Build history of the part. All positions in model axes, mm. A direction names the side the tool comes from. Give positions to 0.01 mm unless a question says otherwise; leave off trailing zeros. Loops run counter-clockwise (first coordinate to the right, second up) from the corner with the lowest first, then second, coordinate; pieces in that order, holes last. Notation, with made-up numbers: (84, 85.25) -> (89, 85.25) arc R23 cw to (89, 124.25) -> close; hole circle Ø2 at (7.25, -17.75). An arc over 180 degrees is marked (long way). One line per question, with ' | ' between items. Start each with the question number.
(1) Flat gauge pins, fed straight in: pin 1 Ø5 at (y, z) = (-27.5, 126.5) entering from +X; pin 2 Ø1 at (x, z) = (-9.5, 86.5) entering from +Y; pin 3 Ø1 at (x, z) = (6, 26.5) entering from -Y; pin 4 Ø21.5 at (x, y) = (0, 0) entering from -Z. Where does each tip first touch, or does it go through?
(2) Drill centre lines: L1, parallel to Y at x = 0, z = 6; L2, parallel to Z at x = -7.5, y = 23.5; L3, parallel to X at y = -15.5, z = 70.5. Where is each one in solid material? Low to high. Write a range as from..to.
(3) Slice it at C-C, the plane z = 54. Write the cut outline in (x, y), then the cut area to 3 significant figures.
(4) Mould opens along X. For faces 1 (the face through (-1, -10, 0)), 2 (the face through (-2.798, 8.885, 10.14)), 3 (the face through (47.69, -15.02, 51.76)) say: pulls with the +X half, pulls with the -X half, needs draft (parallel to the pull), parting line crosses it, or undercut.
(5) Slice it at B-B, the plane y = 41. Write the cut outline in (x, z), then the cut area to 3 significant figures.
(6) Slice it at A-A, the plane x = -43. Write the cut outline in (y, z), then the cut area to 3 significant figures.
(7) 3-axis set-ups, long thin cutter, end or side, ignore diameter. For faces 4 (the face through (0, 0, 150)), 5 (the face through (10, 11, 130)): which of +Z, -Z, +X, -X, +Y, -Y reach the whole face in a straight line?
Autodesk Inventor part; units mm, degrees
ref_plane "YZ Plane" through (0, 0, 0) normal (1, 0, 0) x (0, 1, 0)
ref_plane "XZ Plane" through (0, 0, 0) normal (0, 1, 0) x (-1, 0, 0)
ref_plane "XY Plane" through (0, 0, 0) normal (0, 0, 1) x (1, 0, 0)
sketch "Sketch1" plane through (0, 0, 0) normal (0, 1, 0) x (-1, 0, 0)
  line L0 (0, 0) -> (0, 150)
  line L1 (0, 150) -> (-14, 150)
  line L2 (-14, 150) -> (-14, 130)
  line L3 (-14, 130) -> (-47.5, 130)
  line L4 (-47.5, 130) -> (-47.5, 105)
  line L5 (-47.5, 105) -> (-50, 105)
  line L6 (-50, 105) -> (-50, 0)
  line L7 (-50, 0) -> (0, 0)
  dimension "d0" = 20
  dimension "d1" = 130
  dimension "d2" = 95
  dimension "d3" = 100
  dimension "d4" = 25
  dimension "d5" = 28
revolve "Revolution1" add sketch "Sketch1" angle 360 about axis through (0, 0, 0) along (0, 0, 1)
sketch "Sketch2" plane through (0, 0, 0) normal (0, 0, -1) x (-1, 0, 0)
  point P0 (0, 0)
hole "Hole1" at (0, 0, 0) direction (0, 0, 1) diameter 18.631 depth 20 tip angle 118
properties part number "Pulse compensator"
Final values:
1) pin 1: x = 40.39 | pin 2: y = 49.18 | pin 3: y = -49.7 | pin 4: z = 0
2) L1: -50..-9.32, 9.32..50 | L2: 0..130 | L3: -47.54..47.54
3) outline: circle Ø100 at (0, 0) | area: 7,850 mm2
4) face 1: needs draft | face 2: undercut | face 3: parting line crosses it
5) outline: (-28.62, 0) -> (28.62, 0) -> (28.62, 105) -> (23.98, 105) -> (23.98, 130) -> (-23.98, 130) -> (-23.98, 105) -> (-28.62, 105) -> close | area: 7,210 mm2
6) outline: (-25.51, 0) -> (25.51, 0) -> (25.51, 105) -> (20.18, 105) -> (20.18, 130) -> (-20.18, 130) -> (-20.18, 105) -> (-25.51, 105) -> close | area: 6,370 mm2
7) face 4: +Z, +X, -X, +Y, -Y | face 5: +Z
